```python
from build123d import *

# Parameters (mm, degrees)
F3_DEPTH = 127
F1_W     = 127
F1_H     = 127
F1_R     = 38.1
F4_DEPTH = 194.818
F5_DEPTH = 63.5
F6_DEPTH = 281.432
F7_DEPTH = 672.592
F0_W     = 63.5
F0_H     = 63.5
F8_DEPTH = 261.874


with BuildPart() as f3:
    # F2 (on Right) → F3 (new body, symmetric)
    with BuildSketch(Plane.YZ):
        Polygon((-101.6, -127), (101.6, -127), (101.6, 127), align=None)
    extrude(amount=F3_DEPTH, both=True)

    # F1 (on Top) → F4 (cut)
    with BuildSketch(Plane.XY):
        with Locations((0, 12.7)):
            Rectangle(F1_W, F1_H)
        with Locations((0, 12.7)):
            Circle(F1_R, mode=Mode.SUBTRACT)
    extrude(amount=F4_DEPTH, mode=Mode.SUBTRACT)

    # F1 (on Top) → F5 (cut)
    with BuildSketch(Plane.XY):
        with Locations((0, 12.7)):
            Rectangle(F1_W, F1_H)
        with Locations((0, 12.7)):
            Circle(F1_R, mode=Mode.SUBTRACT)
    extrude(amount=-F5_DEPTH, mode=Mode.SUBTRACT)

    # F1 (on Top) → F6 (cut)
    with BuildSketch(Plane.XY):
        with Locations((0, 12.7)):
            Circle(F1_R)
    extrude(amount=-F6_DEPTH, mode=Mode.SUBTRACT)

    # F1 (on Top) → F7 (cut)
    with BuildSketch(Plane.XY):
        with Locations((0, 12.7)):
            Circle(F1_R)
    extrude(amount=F7_DEPTH, mode=Mode.SUBTRACT)

    # F0 (on Front) → F8 (cut)
    with BuildSketch(Plane.XZ):
        with Locations((0, 19.05)):
            Rectangle(F0_W, F0_H)
    extrude(amount=-F8_DEPTH, mode=Mode.SUBTRACT)


solid = f3.part
```
The listing builds one solid part. Answer for the finished solid, in the listing's coordinates (mm). A direction names the side the tool comes from. Give positions to 0.01 mm unless a question says otherwise; leave off trailing zeros. Write each loop counter-clockwise with the first axis right and the second up, starting at its lowest first coordinate (ties: lowest second). Pieces come first, ordered by that corner, then holes. Notation, with made-up numbers: M 65,-19 L 73,-19 A9 cw 73,-10 Z; hole C 24,-5.75 d5. An arc over 180 degrees is marked long. Write each question's results on one line, items separated by ' | '.
Q1. Consider L1, parallel to X at y = 27, z = -9; L2, parallel to Z at x = -3, y = 67.5; L3, parallel to Y at x = 0, z = -98. Determine where each line is inside the solid, lowest interval first. Write a range as from..to.
Output values:
L1: -127..-63.5, 63.5..127 | L2: -127..-63.5 | L3: -78.4..-25.4, 50.8..101.6
Q2. For a pull along Z with two mould halves and no side action, classify faces 4 (the flat face through (30, -24, -127)), 5 (the flat face through (0, 89, -12.7)), 6 (the flat face through (-63.5, 40, -21)) as released by +Z, released by -Z, zero draft, split by the parting line, or undercut.
Output values:
face 4: released by -Z | face 5: undercut | face 6: zero draft
Q3. Section C-C, the plane y = -44 is taken. Write down the section's boundary in (x, z).
Output values:
outline: M -127,-127 L 127,-127 L 127,-55 L 63.5,-55 L 63.5,-63.5 L -63.5,-63.5 L -63.5,-55 L -127,-55 Z
Q4. A tool of negligible diameter and unlimited length cuts with its end or side. For faces 1 (the flat face through (27, -15, -63.5)), 2 (the flat face through (0, 89, 50.8)), 3 (the flat face through (86.445, 1.422, 1.778)), from which of +Z, -Z, +X, -X, +Y, -Y can it reach the whole face along a straight path? Write none if from no direction.
Output values:
face 1: +Z, -Y | face 2: +Y, -Y | face 3: +Z, +X, -X, -Y
Q5. Flat-ended cylindrical pins translate along their axes: P1, Ø5, axis at x = 69, z = 0.5, coming from the -Y side; P2, Ø1, axis at x = 4, z = -45.5, coming from the -Y side. Find the tip coordinate at first contact, or state that the pin passes through.
Output values:
P1: y = -1.6 | P2: y = 76.2
Q6. Section A-A, the plane x = 0 is taken. Write down the section's boundary in (y, z).
Output values:
outline: M -101.6,-127 L -25.4,-127 L -25.4,-63.5 L -50.8,-63.5 Z; M 50.8,-127 L 101.6,-127 L 101.6,-12.7 L 76.2,-12.7 L 76.2,-63.5 L 50.8,-63.5 Z; M 76.2,50.8 L 101.6,50.8 L 101.6,127 L 76.2,95.25 Z
Q7. Section D-D, the plane z = -110 is taken. Write down the section's boundary in (x, y).
Output values:
outline: M -127,-88 L 127,-88 L 127,101.6 L -127,101.6 Z; hole C 0,12.7 d76.2
Q8. Section B-B, the plane z = -2.5 is taken. Write down the section's boundary in (x, y).
Output values:
outline: M -127,-2 L -63.5,-2 L -63.5,76.2 L -31.75,76.2 L -31.75,101.6 L -127,101.6 Z; M 31.75,76.2 L 63.5,76.2 L 63.5,-2 L 127,-2 L 127,101.6 L 31.75,101.6 Z
